Could you check a few things on this model? Use its own coordinates, in mm. A direction names the side the tool comes from. Coordinates: 2 decimals unless noted, no trailing zeros. Order: outer loops, then holes, each group sorted by start corner. A loop starts at its lowest first (then second) coordinate and runs counter-clockwise, first axis right, second up. Notation, with made-up numbers: (-27.5, 29.5) -> (-7.5, 29.5) arc R31 cw to (-7.5, 55.5) -> close; hole circle Ø8 at (85, -15). An arc over 180 degrees is marked (long way). Use a Markdown table: item, result. Add a question column.
1) If we section it at C-C (z = 21): Write out the boundary of the cut face in (x, y).
2) Will these pins go through, and if not, where does the flat tip stop? pin 1 Ø4.5 at (x, y) = (-59, -15) entering from +Z; pin 2 Ø1 at (x, y) = (12, -16) entering from +Z; pin 3 Ø5 at (x, z) = (46.5, 23) entering from -Y.
3) If we section it at D-D (x = 15): Write out the boundary of the cut face in (y, z), plus the area to 3 significant figures.
4) If we section it at B-B (x = -59): Write out the boundary of the cut face in (y, z), plus the area to 3 significant figures.
5) If we section it at A-A (y = -15): Write out the boundary of the cut face in (x, z), plus the area to 3 significant figures.
6) Which directions (+Z, -Z, +X, -X, +Y, -Y) give clear straight access to the entire face, cutting with the end or side of a thin tool? Please do faces 4 (the flat face through (1, -6, 21)), 5 (the flat face through (-1, 0, 17)).
7) Thinking about a two-plate mould opening in X: for faces 1 (the flat face through (-1, -12, 0)), 2 (the cylindrical face through (61.747, -2.958, 19.629)), 3 (the flat face through (-65.5, -4, 9)), which applies, +X half, -X half, draft (parallel to the pull), parting line (faces both ways), or undercut?
8) If I drill on L1, parallel to X at y = -15.25, z = 5; L2, parallel to Z at x = -59, y = -3.8; L3, parallel to Y at x = 59, z = 4.1, over which ranges is the centre line in solid material (lowest first)? Write a range as [from, to].
```python
from build123d import *

# Parameters (mm, degrees)
SKETCH1_W                = 131
SKETCH1_H                = 25
EXTRUDE1_DEPTH           = 6
SKETCH2_W                = 131
SKETCH2_H                = 35
EXTRUDE2_DEPTH           = 6
M5_CLEARANCE_HOLE1_D     = 5.5
M5_CLEARANCE_HOLE1_DEPTH = 10
M5_CLEARANCE_HOLE1_TIP   = 1.652366702
M5_CLEARANCE_HOLE2_D     = 5.5
M5_CLEARANCE_HOLE2_DEPTH = 10
M5_CLEARANCE_HOLE2_TIP   = 1.652366702


with BuildPart() as part:
    # Sketch1 → Extrude1 (new body)
    with BuildSketch(Plane.XY):
        with Locations((0, -12.5)):
            Rectangle(SKETCH1_W, SKETCH1_H)
    extrude(amount=EXTRUDE1_DEPTH)

    # Sketch2 → Extrude2 (add)
    with BuildSketch(Plane(origin=(0, 0, 0), x_dir=(-1, 0, 0), z_dir=(0, 1, 0))):
        with Locations((0, 17.5)):
            Rectangle(SKETCH2_W, SKETCH2_H)
    extrude(amount=-EXTRUDE2_DEPTH)

    # M5 Clearance Hole1
    with Locations(Plane.XY.offset(6)):
        with Locations((59, -15), (-59, -15)):
            Hole(M5_CLEARANCE_HOLE1_D / 2, depth=M5_CLEARANCE_HOLE1_DEPTH)
            with Locations((0, 0, -(M5_CLEARANCE_HOLE1_DEPTH + M5_CLEARANCE_HOLE1_TIP / 2))):  # 118° drill point
                Cone(0, M5_CLEARANCE_HOLE1_D / 2, M5_CLEARANCE_HOLE1_TIP, mode=Mode.SUBTRACT)

    # M5 Clearance Hole2
    with Locations(Plane(origin=(0.415083287, -6, 44.50809769), x_dir=(1, 0, 0), z_dir=(0, -1, 0))):
        with Locations((58.584916713, -25), (-59.415083287, -25)):
            Hole(M5_CLEARANCE_HOLE2_D / 2, depth=M5_CLEARANCE_HOLE2_DEPTH)
            with Locations((0, 0, -(M5_CLEARANCE_HOLE2_DEPTH + M5_CLEARANCE_HOLE2_TIP / 2))):  # 118° drill point
                Cone(0, M5_CLEARANCE_HOLE2_D / 2, M5_CLEARANCE_HOLE2_TIP, mode=Mode.SUBTRACT)


solid = part.part
```
Answer sheet:
| question | item | result |
|---|---|---|
| 1 | outline | (-65.5, -6) -> (-61.31, -6) -> (-61.31, 0) -> (-65.5, 0) -> close; (-56.69, -6) -> (56.69, -6) -> (56.69, 0) -> (-56.69, 0) -> close; (61.31, -6) -> (65.5, -6) -> (65.5, 0) -> (61.31, 0) -> close |
| 2 | pin 1 | through |
| 2 | pin 2 | z = 6 |
| 2 | pin 3 | y = -6 |
| 3 | outline | (-25, 0) -> (0, 0) -> (0, 35) -> (-6, 35) -> (-6, 6) -> (-25, 6) -> close |
| 3 | area | 324 mm2 |
| 4 | outline | (-25, 0) -> (-17.75, 0) -> (-17.75, 6) -> (-25, 6) -> close; (-12.25, 0) -> (0, 0) -> (0, 16.76) -> (-6, 16.76) -> (-6, 6) -> (-12.25, 6) -> close; (-6, 22.26) -> (0, 22.26) -> (0, 35) -> (-6, 35) -> close |
| 4 | area | 258 mm2 |
| 5 | outline | (-65.5, 0) -> (-61.75, 0) -> (-61.75, 6) -> (-65.5, 6) -> close; (-56.25, 0) -> (56.25, 0) -> (56.25, 6) -> (-56.25, 6) -> close; (61.75, 0) -> (65.5, 0) -> (65.5, 6) -> (61.75, 6) -> close |
| 5 | area | 720 mm2 |
| 6 | face 4 | +Z, +X, -X, -Y |
| 6 | face 5 | +Z, -Z, +X, -X, +Y |
| 7 | face 1 | draft |
| 7 | face 2 | undercut |
| 7 | face 3 | -X half |
| 8 | L1 | [-65.5, -61.74], [-56.26, 56.26], [61.74, 65.5] |
| 8 | L2 | [0, 16.76], [22.26, 35] |
| 8 | L3 | [-25, -17.75], [-12.25, 0] |
